For this review, use the dimensioned drawing (mm, ordinates from the lowest corner) and the shaded views. A direction names the side the tool comes from. Coordinates: 2 decimals unless noted, no trailing zeros. Order: outer loops, then holes, each group sorted by start corner. A loop starts at its lowest first (then second) coordinate and runs counter-clockwise, first axis right, second up. Notation, with made-up numbers: (75.25, -35) -> (82.25, -35) arc R21 cw to (82.25, -2) -> close; hole circle Ø2 at (51.25, 29). An arc over 180 degrees is marked (long way). Return JSON: item names as keys, results as strings. Group by question number.
Item 1: Take a section at B-B (y = 10). Write out the cut boundary in (x, z).
Item 2: Take a section at A-A (z = 12.5). Write out the cut boundary in (x, y), then the cut area to 3 significant figures.
Item 3: For line 1 along Y through (x, z) = (2.3, 34); line 2 along X through (y, z) = (4, 13); line 3 along X through (y, z) = (3, 39), list the stretches that pass through material, from the lowest coordinate up.
Item 4: Take a section at C-C (z = 34). Write out the cut boundary in (x, y), then the cut area to 3 significant figures.
Item 5: Machinability: for the marked faces 1, 2 and 3, which of the approach directions +Z, -Z, +X, -X, +Y, -Y give a long, thin tool a straight path to every point of the face, cutting with its end or side? Answer none if there is none.
Item 6: Draft analysis for pull direction X (two halves, no side actions). For the marked faces 4, 5, 6 and 7, state which applies: +X half, -X half, draft (parallel to the pull), parting line (faces both ways), or undercut.
Item 7: Take a section at D-D (x = 28). Write out the cut boundary in (y, z), then the cut area to 4 significant figures.
Item 8: Insertion check: pin 1 (5 mm diameter, centred on y = 10, z = 34, fed in from +X); pin 2 (8 mm diameter, centred on y = 8.5, z = 37.5, fed in from +X); pin 3 (3 mm diameter, centred on x = 57, y = 14, fed in from +Z). Each pin has a flat end and moves straight along its axis. Give the tip position at first contact, or say it passes through.
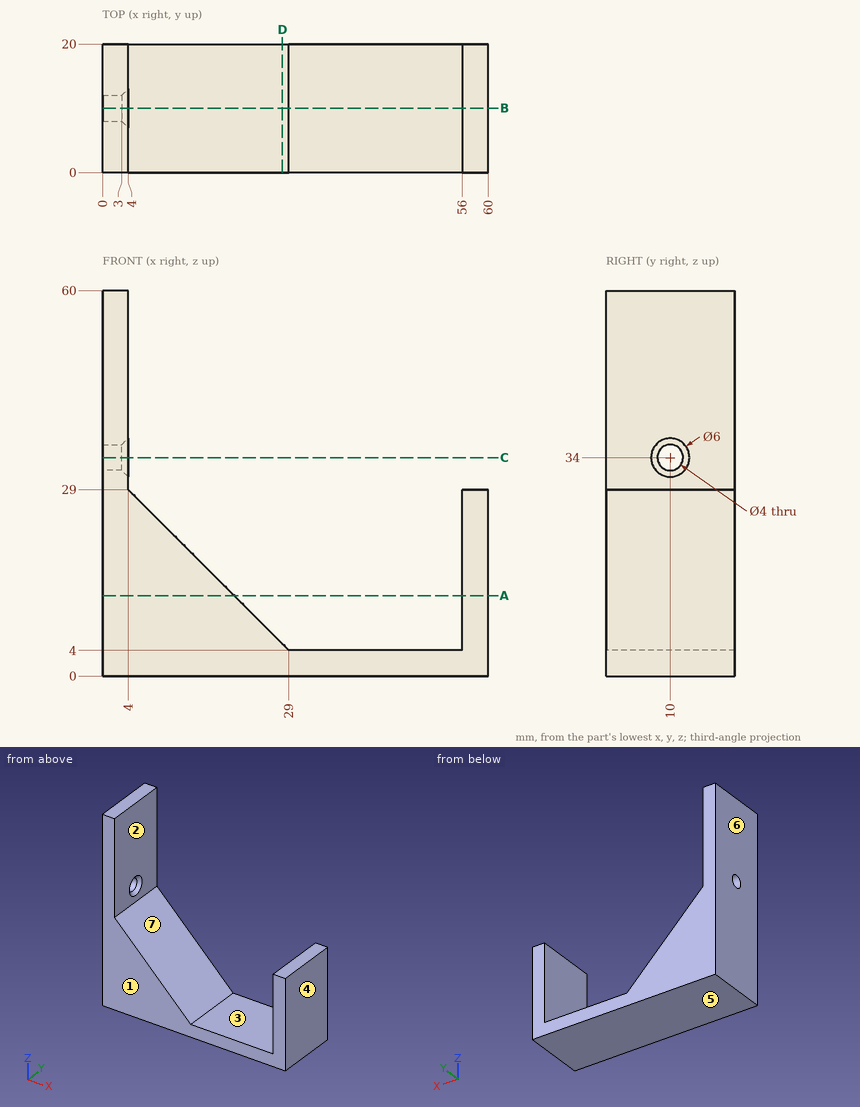
Findings below:
{
 "1": {"outline": "(0, 0) -> (60, 0) -> (60, 29) -> (56, 29) -> (56, 4) -> (29, 4) -> (4, 29) -> (4, 31) -> (3, 32) -> (0, 32) -> close; (0, 36) -> (3, 36) -> (4, 37) -> (4, 60) -> (0, 60) -> close"},
 "2": {"outline": "(0, 0) -> (20.5, 0) -> (20.5, 20) -> (0, 20) -> close; (56, 0) -> (60, 0) -> (60, 20) -> (56, 20) -> close", "area": "490 mm2"},
 "3": {"line 1": "y = 0 to 8, 12 to 20", "line 2": "x = 0 to 20, 56 to 60", "line 3": "x = 0 to 4"},
 "4": {"outline": "(0, 0) -> (4, 0) -> (4, 7) -> (3, 8) -> (0, 8) -> close; (0, 12) -> (3, 12) -> (4, 13) -> (4, 20) -> (0, 20) -> close", "area": "63.0 mm2"},
 "5": {"face 1": "+Z, -Z, +X, -X, -Y", "face 2": "+Z, +X, +Y, -Y", "face 3": "+Z, +Y, -Y"},
 "6": {"face 4": "+X half", "face 5": "draft", "face 6": "-X half", "face 7": "undercut"},
 "7": {"outline": "(0, 0) -> (20, 0) -> (20, 5) -> (0, 5) -> close", "area": "100.0 mm2"},
 "8": {"pin 1": "stops at x = 3.5", "pin 2": "stops at x = 4", "pin 3": "stops at z = 29"}
}
